from build123d import *

# Parameters (mm, degrees)
F0_R      = 3.175
F1_DEPTH  = 152.4
F3_R      = 3.175
F3_R_2    = 2.667
F4_DEPTH  = 0.7366
F6_R      = 3.175
F6_R_2    = 2.667
F7_DEPTH  = 0.7366
F9_R      = 3.175
F9_R_2    = 2.667
F10_DEPTH = 0.7366
F12_R     = 3.175
F12_R_2   = 2.667
F13_DEPTH = 0.7366


with BuildPart() as f1:
    # F0 (on Right) → F1 (new body)
    with BuildSketch(Plane.YZ):
        Circle(F0_R)
    extrude(amount=F1_DEPTH)

    # F3 (on offset) → F4 (cut)
    with BuildSketch(Plane.YZ.offset(138.1125)):
        Circle(F3_R)
        Circle(F3_R_2, mode=Mode.SUBTRACT)
    extrude(amount=-F4_DEPTH, mode=Mode.SUBTRACT)

    # F6 (on offset) → F7 (cut)
    with BuildSketch(Plane(origin=(14.2875, 0, 0), x_dir=(0, 1, 0), z_dir=(-1, 0, 0))):
        Circle(F6_R)
        Circle(F6_R_2, mode=Mode.SUBTRACT)
    extrude(amount=F7_DEPTH, mode=Mode.SUBTRACT)

    # F9 (on offset) → F10 (cut)
    with BuildSketch(Plane.YZ.offset(50.8)):
        Circle(F9_R)
        Circle(F9_R_2, mode=Mode.SUBTRACT)
    extrude(amount=-F10_DEPTH, mode=Mode.SUBTRACT)

    # F12 (on offset) → F13 (cut)
    with BuildSketch(Plane.YZ.offset(101.6)):
        Circle(F12_R)
        Circle(F12_R_2, mode=Mode.SUBTRACT)
    extrude(amount=F13_DEPTH, mode=Mode.SUBTRACT)


solid = f1.part
Design review of the part built by this model. Coordinates are the model's own, in mm. A direction names the side the tool comes from. Coordinates: 2 decimals unless noted, no trailing zeros. Order: outer loops, then holes, each group sorted by start corner. A loop starts at its lowest first (then second) coordinate and runs counter-clockwise, first axis right, second up. Notation, with made-up numbers: M -25.5,49.5 L -20.5,49.5 A9 ccw -20.5,64.5 Z; hole C 78.5,33.5 d3. An arc over 180 degrees is marked long. Use a Markdown table: item, result.
(1) Add section A-A (x = 125). Give the boundary of the cut face in (y, z) (3 decimals).
Worked answers:
| item | result |
|---|---|
| outline | C 0,0 d6.35 |
(2) Draft analysis for pull direction X (two halves, no side actions). For faces 3 (the cylindrical face through (31.93, -0.69, -3.1)), 4 (the flat face through (13.551, -2, -2)), 5 (the flat face through (152.4, 0, 0)), 6 (the flat face through (0, 0, 0)), state which applies: released by +X, released by -X, zero draft, split by the parting line, or undercut.
Worked answers:
| item | result |
|---|---|
| face 3 | zero draft |
| face 4 | undercut |
| face 5 | released by +X |
| face 6 | released by -X |
(3) Wall thickness on probe 1 along X at (y, z) = (-2.75, 1.5); probe 2 along Y at (x, z) = (105, -1.75); probe 3 along Z at (x, y) = (106, 0.25): over which ranges is each line inside the solid? List them lowest first.
Worked answers:
| item | result |
|---|---|
| probe 1 | x = 0 to 13.55, 14.29 to 50.06, 50.8 to 101.6, 102.34 to 137.38, 138.11 to 152.4 |
| probe 2 | y = -2.65 to 2.65 |
| probe 3 | z = -3.17 to 3.17 |
(4) For P1, Ø3, axis at x = 61.5, z = 2.5, coming from the -Y side, flat-tipped, find the tip position at first contact; note if it passes through.
Worked answers:
| item | result |
|---|---|
| P1 | stops at y = -3.01 |
(5) For faces 1 (the flat face through (50.8, -2, 2)), 2 (the cylindrical face through (145.16, -0.69, -3.1)), list the 3-axis set-ups (+Z, -Z, +X, -X, +Y, -Y) from which the entire face can be reached by the end or side of a thin tool; tool diameter is ignored.
Worked answers:
| item | result |
|---|---|
| face 1 | none |
| face 2 | +X, -X |
